Autodesk Inventor part; units mm, degrees
ref_plane "YZ Plane" through (0, 0, 0) normal (1, 0, 0) x (0, 1, 0)
ref_plane "XZ Plane" through (0, 0, 0) normal (0, 1, 0) x (-1, 0, 0)
ref_plane "XY Plane" through (0, 0, 0) normal (0, 0, 1) x (1, 0, 0)
sketch "草圖1" plane through (0, 0, 0) normal (0, 0, 1) x (1, 0, 0)
  line L0 (0, 0) -> (-25.5595, 13.402) construction
  line L1 (-25.5595, 13.402) -> (9.701, 12.2296) construction
  line L2 (9.701, 12.2296) -> (0, 0) construction
  line L3 (-25.5595, 13.402) -> (0, 0) construction
  line L4 (-26.1399, 12.2949) -> (-0.5805, -1.107)
  line L5 (0.5805, 1.107) -> (-24.979, 14.509)
  arc A0 (-24.979, 14.509) -> (-26.1399, 12.2949) centre (-25.5595, 13.402) ccw
  arc A1 (-0.5805, -1.107) -> (0.5805, 1.107) centre (0, 0) ccw
  line L6 (-25.5595, 13.402) -> (9.701, 12.2296) construction
  line L7 (-25.601, 12.1527) -> (9.6595, 10.9802)
  line L8 (9.7426, 13.4789) -> (-25.5179, 14.6513)
  arc A2 (-25.5179, 14.6513) -> (-25.601, 12.1527) centre (-25.5595, 13.402) ccw
  arc A3 (9.6595, 10.9802) -> (9.7426, 13.4789) centre (9.701, 12.2296) ccw
  line L9 (9.701, 12.2296) -> (0, 0) construction
  line L10 (8.7217, 13.0064) -> (-0.9793, 0.7768)
  line L11 (0.9793, -0.7768) -> (10.6803, 11.4527)
  arc A4 (10.6803, 11.4527) -> (8.7217, 13.0064) centre (9.701, 12.2296) ccw
  arc A5 (-0.9793, 0.7768) -> (0.9793, -0.7768) centre (0, 0) ccw
  point P0 (-12.7797, 6.701)
  point P1 (-7.9292, 12.8158)
  point P2 (4.8505, 6.1148)
  dimension "d0" = 28.86
  dimension "d1" = 35.28
  dimension "d2" = 15.61
  dimension "d3" = 2.5
  dimension "d4" = 2.5
  dimension "d5" = 2.5
extrude "擠出1" add sketch "草圖1" along normal blind 2 contours A2 L7 L5 L10 A5 L4 | A0 L5 L7 A2 | A5 L10 L5 A1 | L8 A4 L10 L7 L5 A0 | A1 L5 L10 L7 A3 L11 | A3 L7 L10 A4
sketch "草圖2" plane through (0, 0, 2) normal (0, 0, 1) x (1, 0, 0)
  arc A0 (10.6803, 11.4527) -> (9.7426, 13.4789) centre (9.701, 12.2296) ccw
  arc A1 (-25.5179, 14.6513) -> (-26.1399, 12.2949) centre (-25.5595, 13.402) ccw
  arc A2 (-0.5805, -1.107) -> (0.9793, -0.7768) centre (0, 0) ccw
  circle A3 centre (0, 0) radius 0.625
  circle A4 centre (9.701, 12.2296) radius 0.625
  circle A5 centre (-25.5595, 13.402) radius 0.625
  dimension "d8" = 1.25
  dimension "d9" = 1.25
  dimension "d10" = 1.25
extrude "擠出2" cut sketch "草圖2" against normal blind 2
sketch "草圖4" plane through (0, 0, 2) normal (0, 0, 1) x (1, 0, 0)
  circle A0 centre (-25.5595, 13.402) radius 0.625
  line L0 (-0.3361, 1.5877) -> (-20.1387, 11.971)
  line L1 (-20.1387, 11.971) -> (7.1799, 11.0627)
  line L2 (9.7426, 13.4789) -> (-25.5179, 14.6513)
  arc A1 (-25.5179, 14.6513) -> (-26.1399, 12.2949) centre (-25.5595, 13.402) ccw
  line L3 (-26.1399, 12.2949) -> (-0.5805, -1.107)
  line L4 (-5.5082, 13.986) -> (-6.7973, 11.5274)
  line L5 (-9.4919, 6.3884) -> (-10.6529, 4.1744)
extrude "擠出3" add sketch "草圖4" along normal blind 4
sketch "草圖5" plane through (0, 0, 6) normal (0, 0, 1) x (1, 0, 0)
  circle A0 centre (-21.6744, 19.594) radius 6
  point P0 (0, 0)
  dimension "d17" = 12
extrude "擠出4" cut sketch "草圖5" against normal blind 40
sketch "草圖7" plane through (0, 0, 6) normal (0, 0, 1) x (1, 0, 0)
  arc A0 (-25.0533, 14.6358) -> (-18.6323, 14.4223) centre (-21.6744, 19.594) ccw
  line L0 (-25.0533, 14.6358) -> (-25.5179, 14.6513)
  arc A1 (-19.7698, 13.9043) -> (-16.0409, 17.5291) centre (-21.6744, 19.594) ccw
  arc A2 (-18.8815, 13.6327) -> (-15.4885, 17.3418) centre (-21.6744, 19.594) ccw
  line L1 (-16.0409, 17.5291) -> (-15.4885, 17.3418)
  line L2 (-19.7698, 13.9043) -> (-18.8815, 13.6327)
  point P0 (0, 0)
extrude "擠出5" add sketch "草圖7" against normal blind 6
sketch "草圖8" plane through (0, 0, 6) normal (0, 0, 1) x (1, 0, 0)
  line L0 (-36.1611, 22.8385) -> (7.9162, 22.8385)
  line L1 (7.9162, 22.8385) -> (7.9162, -4.1508)
  line L2 (7.9162, -4.1508) -> (-36.1611, -4.1508)
  line L3 (-36.1611, -4.1508) -> (-36.1611, 22.8385)
  point P0 (0, 0)
extrude "擠出6" cut sketch "草圖8" against normal blind 1.5
sketch "草圖9" plane through (0, 0, 0) normal (0, 0, -1) x (-1, 0, 0)
  line L0 (-9.7426, 13.4789) -> (17.6433, 14.3894)
  arc A0 (-9.7426, 13.4789) -> (-10.6803, 11.4527) centre (-9.701, 12.2296) ccw
  line L1 (-0.9793, -0.7768) -> (-10.6803, 11.4527)
  arc A1 (-0.9793, -0.7768) -> (0.5805, -1.107) centre (0, 0) ccw
  line L2 (26.1399, 12.2949) -> (0.5805, -1.107)
  arc A2 (26.1399, 12.2949) -> (25.5179, 14.6513) centre (25.5595, 13.402) ccw
  line L3 (25.0533, 14.6358) -> (25.5179, 14.6513)
  arc A3 (16.0409, 17.5291) -> (25.0533, 14.6358) centre (21.6744, 19.594) ccw
  line L4 (16.0409, 17.5291) -> (15.4885, 17.3418)
  arc A4 (15.4885, 17.3418) -> (17.6433, 14.3894) centre (21.6744, 19.594) ccw
  line L5 (-7.1799, 11.0627) -> (0.3361, 1.5877)
  line L6 (20.1387, 11.971) -> (-7.1799, 11.0627)
  line L7 (0.3361, 1.5877) -> (20.1387, 11.971)
  circle A5 centre (25.5595, 13.402) radius 0.625
  circle A6 centre (0, 0) radius 0.625
  circle A7 centre (-9.701, 12.2296) radius 0.625
extrude "擠出7" cut sketch "草圖9" against normal blind 1.5
sketch "草圖6" plane through (0, 0, 2) normal (0, 0, 1) x (1, 0, 0)
  arc A0 (-26.0169, 18.4563) -> (-17.0179, 18.323) centre (-21.5174, 18.3896) ccw
  line L0 (-26.0169, 18.4563) -> (-17.0179, 18.323)
  dimension "d20" = 9
sketch "草圖3" plane through (0, 0, 2) normal (0, 0, 1) x (1, 0, 0)
  line L0 (9.7426, 13.4789) -> (-25.5179, 14.6513)
  arc A0 (-25.5179, 14.6513) -> (-26.1399, 12.2949) centre (-25.5595, 13.402) ccw
  line L1 (-26.1399, 12.2949) -> (-0.5805, -1.107)
  line L2 (-25.5595, 17.902) -> (-25.5595, 8.902)
  arc A1 (-22.3114, 10.2875) -> (-21.1974, 14.5076) centre (-25.5595, 13.402) ccw
  arc A2 (-25.5595, 17.902) -> (-25.5595, 8.902) centre (-25.5595, 13.402) ccw
properties part number "1-1"
Can you work these out from the model? Positions are in its coordinate system, mm. A direction names the side the tool comes from. Give positions to 0.01 mm unless a question says otherwise; leave off trailing zeros. Write each loop counter-clockwise with the first axis right and the second up, starting at its lowest first coordinate (ties: lowest second). Pieces come first, ordered by that corner, then holes. Notation, with made-up numbers: (46, 57) -> (74, 57) arc R36 cw to (74, 92) -> close; hole circle Ø8 at (47.5, -38). An arc over 180 degrees is marked (long way). Answer as a JSON object with one key per item and string values. Group by question number.
Item 1: Please list where these lines run through material, in increasing order: line 1 (Y direction, x = -13.5, z = 2.3); line 2 (Z direction, x = 0, y = 12.75); line 3 (Y direction, x = -19, z = 4.2). Write a range as [from, to].
Item 2: I'm going to push flat-ended pins straight in: P1, Ø2, axis at x = -25.56, y = 13.4, coming from the +Z side; P2, Ø1.4, axis at x = 0, y = 0, coming from the +Z side. Where does each tip first touch, or does it pass through?
Item 3: Suppose I cut it at A-A (x = -6). Please give me the cut outline in (y, z).
Item 4: Suppose I cut it at D-D (y = 0). Please give me the cut outline in (x, z) (1 decimal).
Item 5: Suppose I cut it at B-B (y = 5). Please give me the cut outline in (x, z).
Item 6: For faces 1 (the face through (-10.064, 5.297, 3.232)), 2 (the face through (-15, 12, 4.5)), 3 (the face through (3.474, 6.391, 1.746)), which set-ups out of +Z, -Z, +X, -X, +Y, -Y let a thin tool reach every point of the face, with its end or its side?
Findings:
{
 "1": {"line 1": "y = [5.67, 8.49], [11.75, 14.25]", "line 2": "z = [1.5, 2]", "line 3": "y = [8.55, 11.37], [11.93, 14.22]"},
 "2": {"P1": "stops at z = 4.5", "P2": "stops at z = 2"},
 "3": {"outline": "(1.73, 1.5) -> (4.56, 1.5) -> (4.56, 2) -> (1.73, 2) -> close; (11.5, 1.5) -> (14, 1.5) -> (14, 4.5) -> (13.05, 4.5) -> (13.05, 2) -> (11.5, 2) -> close"},
 "4": {"outline": "(-2.7, 1.5) -> (-0.6, 1.5) -> (-0.6, 2) -> (-2.7, 2) -> close; (0.6, 1.5) -> (1.6, 1.5) -> (1.6, 2) -> (0.6, 2) -> close"},
 "5": {"outline": "(-12.23, 1.5) -> (-6.84, 1.5) -> (-6.84, 2) -> (-10.22, 2) -> (-10.22, 4.5) -> (-12.23, 4.5) -> close; (2.37, 1.5) -> (5.56, 1.5) -> (5.56, 2) -> (2.37, 2) -> close"},
 "6": {"face 1": "+Z, +X, -Y", "face 2": "+Z, +X, -X, +Y, -Y", "face 3": "+Z, -Z"}
}
